Build history of the part. All positions in model axes, mm. Round coordinates to 2 decimals unless told otherwise and drop trailing zeros. Write each loop counter-clockwise with the first axis right and the second up, starting at its lowest first coordinate (ties: lowest second). Pieces come first, ordered by that corner, then holes. Notation, with made-up numbers: (6, 82.25) -> (29, 82.25) arc R17 ccw to (29, 111.25) -> close; hole circle Ø5 at (25.5, 6.5). An arc over 180 degrees is marked (long way). One line per question, with ' | ' between items.
from build123d import *

# Parameters (mm, degrees)
F0_R     = 50.8
F0_R_2   = 3.175
F1_DEPTH = 6.35
F2_R     = 0.4445


with BuildPart() as f1:
    # F0 (on Front) → F1 (new body)
    with BuildSketch(Plane.XZ):
        Circle(F0_R)
        with Locations((0, -38.1)):
            Circle(F0_R_2, mode=Mode.SUBTRACT)
        with Locations((-38.1, 0)):
            Circle(F0_R_2, mode=Mode.SUBTRACT)
        with Locations((38.1, 0)):
            Circle(F0_R_2, mode=Mode.SUBTRACT)
        with Locations((0, 38.1)):
            Circle(F0_R_2, mode=Mode.SUBTRACT)
    extrude(amount=F1_DEPTH)

    # F2
    f2_edges = [f1.edges().sort_by_distance(p)[0] for p in [
        (-50.8, -6.35, 0),
    ]]
    fillet(f2_edges, radius=F2_R)


solid = f1.part
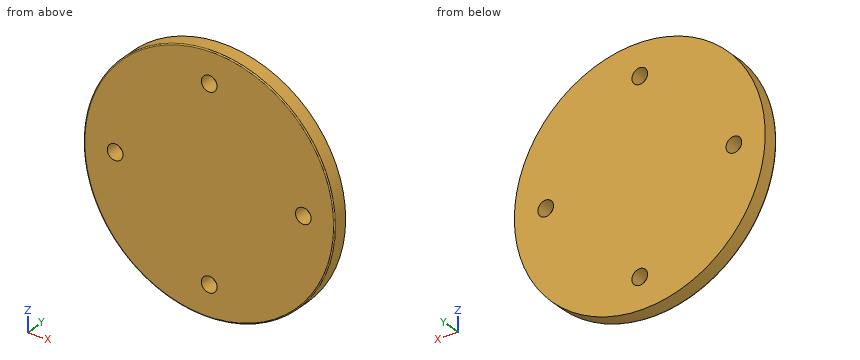
(1) Drop flat-ended pins along their axis: pin 1 (1 mm diameter, centred on x = -26.5, y = -1.5, fed in from -Z); pin 2 (2 mm diameter, centred on x = -38.5, y = -3.5, fed in from -Z). Give the stop position or say it passes through.
Calculated:
pin 1: z = -43.64 | pin 2: z = -34.27
(2) Slice it at C-C (y = -2.25). Write the cut outline in (x, z) (3 decimals), then the cut area to 3 significant figures.
Calculated:
outline: circle Ø101.6 at (0, 0); hole circle Ø6.35 at (-38.1, 0); hole circle Ø6.35 at (0, -38.1); hole circle Ø6.35 at (0, 38.1); hole circle Ø6.35 at (38.1, 0) | area: 7,980 mm2
(3) Wall check: line 1 (Z direction, x = 0, y = -5) (3 decimals); line 2 (Z direction, x = -38.1, y = -3.75) (3 decimals); line 3 (Z direction, x = 41, y = -3). Give the ranges that are in metal, low to high. Write a range as from..to.
Calculated:
line 1: -50.8..-41.275, -34.925..34.925, 41.275..50.8 | line 2: -33.601..-3.175, 3.175..33.601 | line 3: -29.99..-1.29, 1.29..29.99
(4) Slice it at A-A (x = 0). State how many separate pieces and enclosed holes the cut face has, then the cut area to 3 significant figures.
Calculated:
separate pieces: 3 | enclosed holes: 0 | area: 564 mm2
